For this review, use the dimensioned drawing (mm, ordinates from the lowest corner) and the shaded views. A direction names the side the tool comes from. Coordinates: 2 decimals unless noted, no trailing zeros. Loops run counter-clockwise (first coordinate to the right, second up) from the corner with the lowest first, then second, coordinate; pieces in that order, holes last. Notation, with made-up numbers: M 74,26.25 L 119,26.25 A20 ccw 119,55.25 Z; hole C 14.25,29.25 d11. An arc over 180 degrees is marked long. Write item = value, one per line.
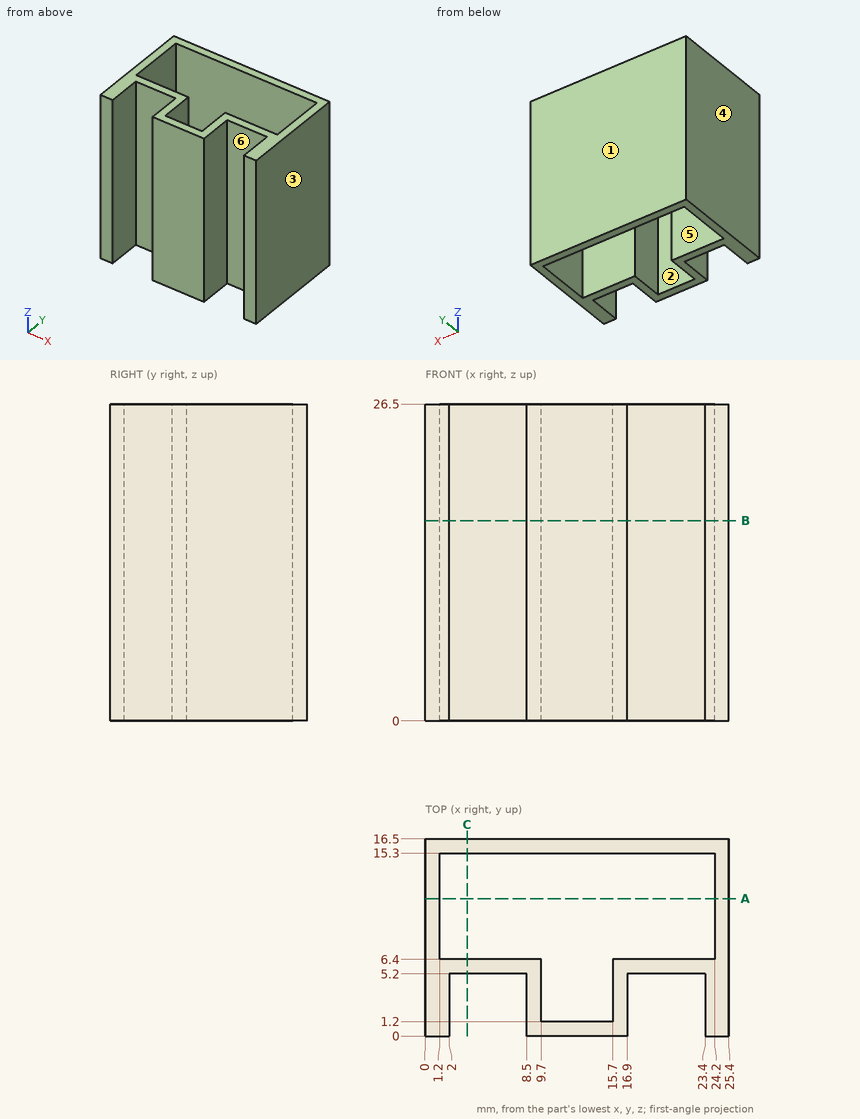
Q1. Machinability: for the marked faces 4, 5 and 6, which of the approach directions +Z, -Z, +X, -X, +Y, -Y give a long, thin tool a straight path to every point of the face, cutting with its end or side? Answer none if there is none.
Solved:
face_4 = +Z, -Z, -X, +Y, -Y
face_5 = +Z, -Z
face_6 = +Z, -Z, -Y
Q2. Add section A-A (y = 11.5). Write out the cut boundary in (x, z).
Solved:
outline = M 0,0 L 1.2,0 L 1.2,26.5 L 0,26.5 Z; M 24.2,0 L 25.4,0 L 25.4,26.5 L 24.2,26.5 Z
Q3. Draft analysis for pull direction Y (two halves, no side actions). For the marked faces 1, 2 and 3, state which applies: +Y half, -Y half, draft (parallel to the pull), parting line (faces both ways), or undercut.
Solved:
face_1 = +Y half
face_2 = undercut
face_3 = draft
Q4. For pin 1 Ø3 at (x, z) = (5.5, 19) entering from -Y, flat-tipped, find the tip position at first contact; note if it passes through.
Solved:
pin_1 = 5.2
Q5. Add section C-C (x = 3.5). Write out the cut boundary in (y, z).
Solved:
outline = M 5.2,0 L 6.4,0 L 6.4,26.5 L 5.2,26.5 Z; M 15.3,0 L 16.5,0 L 16.5,26.5 L 15.3,26.5 Z
Q6. For line 1 along X through (y, z) = (4.25, 22.75); line 2 along X through (y, z) = (8.5, 1.5); line 3 along Y through (x, z) = (6, 6.5), list the stretches that pass through material, from the lowest coordinate up.
Solved:
line_1 = 0 to 2, 8.5 to 9.7, 15.7 to 16.9, 23.4 to 25.4
line_2 = 0 to 1.2, 24.2 to 25.4
line_3 = 5.2 to 6.4, 15.3 to 16.5
Q7. Add section B-B (z = 16.75). Write out the cut boundary in (x, y), and give its area (3 significant figures).
Solved:
outline = M 0,0 L 2,0 L 2,5.2 L 8.5,5.2 L 8.5,0 L 16.9,0 L 16.9,5.2 L 23.4,5.2 L 23.4,0 L 25.4,0 L 25.4,16.5 L 0,16.5 Z; hole M 1.2,6.4 L 9.7,6.4 L 9.7,1.2 L 15.7,1.2 L 15.7,6.4 L 24.2,6.4 L 24.2,15.3 L 1.2,15.3 Z
area = 116 mm²
